Could you check a few things on this drawing? It's one solid part, dimensions in mm from its lowest x, y, z. Give positions to 0.01 mm unless a question says otherwise; leave off trailing zeros. Order: outer loops, then holes, each group sorted by start corner. A loop starts at its lowest first (then second) coordinate and runs counter-clockwise, first axis right, second up. Notation, with made-up numbers: (61, 85) - (115, 85) arc R13 ccw to (115, 105) - close; hole circle Ø11 at (-33.75, 85.5). An arc over 180 degrees is marked (long way). Put each result on its own line as item: value.
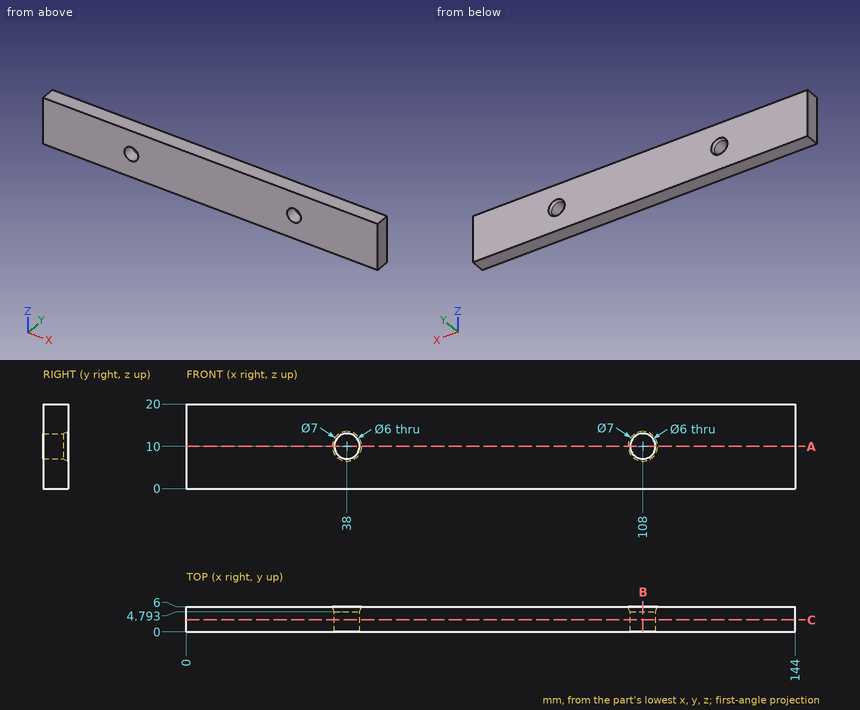
1) Suppose I cut it at A-A, the plane z = 10. List the corners of the cut face in (x, y) for me, and give its area (3 significant figures).
Filled in:
outline: (0, 0) - (35, 0) - (35, 4.79) - (34.5, 6) - (0, 6) - close; (41, 0) - (105, 0) - (105, 4.79) - (104.5, 6) - (41.5, 6) - (41, 4.79) - close; (111, 0) - (144, 0) - (144, 6) - (111.5, 6) - (111, 4.79) - close
area: 791 mm^2
2) Suppose I cut it at C-C, the plane y = 2.85. List the corners of the cut face in (x, z) for me, and give its area (3 significant figures).
Filled in:
outline: (0, 0) - (144, 0) - (144, 20) - (0, 20) - close; hole circle Ø6 at (38, 10); hole circle Ø6 at (108, 10)
area: 2,820 mm^2
3) Suppose I cut it at B-B, the plane x = 108. List the corners of the cut face in (y, z) for me, and give its area (3 significant figures).
Filled in:
outline: (0, 0) - (6, 0) - (6, 6.5) - (4.79, 7) - (0, 7) - close; (0, 13) - (4.79, 13) - (6, 13.5) - (6, 20) - (0, 20) - close
area: 83.4 mm^2
4) If I drill on line 1 (X direction, y = 3.7, z = 10); line 2 (X direction, y = 0.35, z = 12.5); line 3 (Z direction, x = 38, y = 3.6), over which ranges is the centre line in solid material (lowest first)? Write a range as [from, to].
Filled in:
line 1: x = [0, 35], [41, 105], [111, 144]
line 2: x = [0, 36.34], [39.66, 106.34], [109.66, 144]
line 3: z = [0, 7], [13, 20]
